```python
from build123d import *

# Parameters (mm, degrees)
SKETCH1_W                    = 406.4
SKETCH1_H                    = 50.8
EXTRUDE1_DEPTH               = 12.7
SKETCH2_W                    = 12.7
SKETCH2_H                    = 50.8
CUT_EXTRUDE1_DEPTH           = 3.175
SKETCH3_W                    = 44.45
SKETCH3_H                    = 31.75
SKETCH3_W_2                  = 76.2
CUT_EXTRUDE2_DEPTH           = 9.525
FILLET1_R                    = 6.35
SKETCH4_R                    = 2.38125
CUT_EXTRUDE3_DEPTH           = 15.875
SKETCH5_R                    = 3.175
CUT_EXTRUDE4_DEPTH           = 410.673437783
SKETCH6_R                    = 6.7437
CUT_EXTRUDE5_DEPTH           = 410.759551445
CUT_EXTRUDE5_DRAFT           = -41
CUT_EXTRUDE5_PROFILE_2_DEPTH = 410.759551445
CUT_EXTRUDE5_PROFILE_2_DRAFT = -41
CUT_EXTRUDE5_PROFILE_3_DEPTH = 410.759551445
CUT_EXTRUDE5_PROFILE_3_DRAFT = -41
CUT_EXTRUDE5_PROFILE_4_DEPTH = 410.759551445
CUT_EXTRUDE5_PROFILE_4_DRAFT = -41
SKETCH7_R                    = 3.175
CUT_EXTRUDE6_DEPTH           = 15.875
CUT_EXTRUDE7_START           = -15.875
SKETCH8_R                    = 3.175
CUT_EXTRUDE7_DEPTH           = 15.875


with BuildPart() as part:
    # Sketch1 → Extrude1 (new body)
    with BuildSketch(Plane(origin=(0, 0, 0), x_dir=(0, 0, -1), z_dir=(1, 0, 0))):
        with Locations((-203.2, 25.4)):
            Rectangle(SKETCH1_W, SKETCH1_H)
    extrude(amount=EXTRUDE1_DEPTH)

    # Sketch2 → Cut-Extrude1 (cut)
    with BuildSketch(Plane.ZY):
        with Locations((146.05, 25.4)):
            Rectangle(SKETCH2_W, SKETCH2_H)
        with Locations((260.35, 25.4)):
            Rectangle(SKETCH2_W, SKETCH2_H)
    extrude(amount=-CUT_EXTRUDE1_DEPTH, mode=Mode.SUBTRACT)

    # Sketch3 → Cut-Extrude2 (cut)
    with BuildSketch(Plane.ZY):
        with Locations((47.625, 25.4)):
            Rectangle(SKETCH3_W, SKETCH3_H)
        with Locations((104.775, 25.4)):
            Rectangle(SKETCH3_W, SKETCH3_H)
        with Locations((203.2, 25.4)):
            Rectangle(SKETCH3_W_2, SKETCH3_H)
        with Locations((301.625, 25.4)):
            Rectangle(SKETCH3_W, SKETCH3_H)
        with Locations((358.775, 25.4)):
            Rectangle(SKETCH3_W, SKETCH3_H)
    extrude(amount=-CUT_EXTRUDE2_DEPTH, mode=Mode.SUBTRACT)

    # Fillet1
    fillet1_edges = [part.edges().sort_by_distance(p)[0] for p in [
        (4.7625, 9.525, 25.4),
        (4.7625, 41.275, 25.4),
        (4.7625, 41.275, 69.85),
        (4.7625, 9.525, 69.85),
        (4.7625, 41.275, 127),
        (4.7625, 9.525, 127),
        (4.7625, 9.525, 82.55),
        (4.7625, 41.275, 82.55),
        (4.7625, 9.525, 165.1),
        (4.7625, 41.275, 165.1),
        (4.7625, 41.275, 241.3),
        (4.7625, 9.525, 241.3),
        (4.7625, 9.525, 279.4),
        (4.7625, 41.275, 279.4),
        (4.7625, 41.275, 323.85),
        (4.7625, 9.525, 323.85),
        (4.7625, 9.525, 336.55),
        (4.7625, 41.275, 336.55),
        (4.7625, 41.275, 381),
        (4.7625, 9.525, 381),
    ]]
    fillet(fillet1_edges, radius=FILLET1_R)

    # Sketch4 → Cut-Extrude3 (cut)
    with BuildSketch(Plane(origin=(0, 50.8, 0), x_dir=(-1, 0, 0), z_dir=(0, 1, 0))):
        with Locations(Location((-6.35, 19.05, 0), (0, 0, 90))):
            Circle(SKETCH4_R)
        with Locations(Location((-6.35, 133.35, 0), (0, 0, 90))):
            Circle(SKETCH4_R)
        with Locations(Location((-6.35, 273.05, 0), (0, 0, 90))):
            Circle(SKETCH4_R)
        with Locations(Location((-6.35, 387.35, 0), (0, 0, 90))):
            Circle(SKETCH4_R)
    cut_extrude3 = extrude(amount=-CUT_EXTRUDE3_DEPTH, mode=Mode.SUBTRACT)

    # Mirror1: Cut-Extrude3 across plane
    add(cut_extrude3.mirror(Plane.ZX.offset(25.4)), mode=Mode.SUBTRACT)

    # Sketch5 → Cut-Extrude4 (cut, through all)
    with BuildSketch(Plane.ZY.offset(-3.175)):
        with Locations((260.35, 41.275)):
            Circle(SKETCH5_R)
        with Locations((260.35, 9.525)):
            Circle(SKETCH5_R)
        with Locations((146.05, 41.275)):
            Circle(SKETCH5_R)
        with Locations((146.05, 9.525)):
            Circle(SKETCH5_R)
    extrude(amount=-CUT_EXTRUDE4_DEPTH, mode=Mode.SUBTRACT)


with BuildPart() as cut_extrude5_tool:
    # Sketch6 → Cut-Extrude5 (with draft: the straight prism first)
    with BuildSketch(Plane(origin=(12.7, 0, 0), x_dir=(0, 0, -1), z_dir=(1, 0, 0))):
        with Locations((-260.35, 41.275)):
            Circle(SKETCH6_R)
    extrude(amount=-CUT_EXTRUDE5_DEPTH)
    # Cut-Extrude5: the draft: its side faces are tilted about the plane it starts from
    cut_extrude5_sides = [cut_extrude5_tool.faces().sort_by_distance(p)[0] for p in [
        (-192.679775722, 41.275, 267.0937),
    ]]
    draft(cut_extrude5_sides, Plane(origin=(12.7, 0, 0), x_dir=(0, 0, -1), z_dir=(1, 0, 0)), CUT_EXTRUDE5_DRAFT)


with BuildPart() as part_1:
    add(part.part)

    # Cut-Extrude5: cut by cut_extrude5_tool
    add(cut_extrude5_tool.part, mode=Mode.SUBTRACT)


with BuildPart() as cut_extrude5_profile_2_tool:
    # Sketch6 → Cut-Extrude5 profile 2 (with draft: the straight prism first)
    with BuildSketch(Plane(origin=(12.7, 0, 0), x_dir=(0, 0, -1), z_dir=(1, 0, 0))):
        with Locations((-260.35, 9.525)):
            Circle(SKETCH6_R)
    extrude(amount=-CUT_EXTRUDE5_PROFILE_2_DEPTH)
    # Cut-Extrude5 profile 2: the draft: its side faces are tilted about the plane it starts from
    cut_extrude5_profile_2_sides = [cut_extrude5_profile_2_tool.faces().sort_by_distance(p)[0] for p in [
        (-192.679775722, 9.525, 267.0937),
    ]]
    draft(cut_extrude5_profile_2_sides, Plane(origin=(12.7, 0, 0), x_dir=(0, 0, -1), z_dir=(1, 0, 0)), CUT_EXTRUDE5_PROFILE_2_DRAFT)


with BuildPart() as part_2:
    add(part_1.part)

    # Cut-Extrude5 profile 2: cut by cut_extrude5_profile_2_tool
    add(cut_extrude5_profile_2_tool.part, mode=Mode.SUBTRACT)


with BuildPart() as cut_extrude5_profile_3_tool:
    # Sketch6 → Cut-Extrude5 profile 3 (with draft: the straight prism first)
    with BuildSketch(Plane(origin=(12.7, 0, 0), x_dir=(0, 0, -1), z_dir=(1, 0, 0))):
        with Locations((-146.05, 9.525)):
            Circle(SKETCH6_R)
    extrude(amount=-CUT_EXTRUDE5_PROFILE_3_DEPTH)
    # Cut-Extrude5 profile 3: the draft: its side faces are tilted about the plane it starts from
    cut_extrude5_profile_3_sides = [cut_extrude5_profile_3_tool.faces().sort_by_distance(p)[0] for p in [
        (-192.679775722, 9.525, 152.7937),
    ]]
    draft(cut_extrude5_profile_3_sides, Plane(origin=(12.7, 0, 0), x_dir=(0, 0, -1), z_dir=(1, 0, 0)), CUT_EXTRUDE5_PROFILE_3_DRAFT)


with BuildPart() as part_3:
    add(part_2.part)

    # Cut-Extrude5 profile 3: cut by cut_extrude5_profile_3_tool
    add(cut_extrude5_profile_3_tool.part, mode=Mode.SUBTRACT)


with BuildPart() as cut_extrude5_profile_4_tool:
    # Sketch6 → Cut-Extrude5 profile 4 (with draft: the straight prism first)
    with BuildSketch(Plane(origin=(12.7, 0, 0), x_dir=(0, 0, -1), z_dir=(1, 0, 0))):
        with Locations((-146.05, 41.275)):
            Circle(SKETCH6_R)
    extrude(amount=-CUT_EXTRUDE5_PROFILE_4_DEPTH)
    # Cut-Extrude5 profile 4: the draft: its side faces are tilted about the plane it starts from
    cut_extrude5_profile_4_sides = [cut_extrude5_profile_4_tool.faces().sort_by_distance(p)[0] for p in [
        (-192.679775722, 41.275, 152.7937),
    ]]
    draft(cut_extrude5_profile_4_sides, Plane(origin=(12.7, 0, 0), x_dir=(0, 0, -1), z_dir=(1, 0, 0)), CUT_EXTRUDE5_PROFILE_4_DRAFT)


with BuildPart() as part_4:
    add(part_3.part)

    # Cut-Extrude5 profile 4: cut by cut_extrude5_profile_4_tool
    add(cut_extrude5_profile_4_tool.part, mode=Mode.SUBTRACT)

    # Sketch7 → Cut-Extrude6 (cut)
    with BuildSketch(Plane(origin=(0, 0, 0), x_dir=(-1, 0, 0), z_dir=(0, 0, -1))):
        with Locations((-6.35, 41.275)):
            Circle(SKETCH7_R)
        with Locations((-6.35, 9.525)):
            Circle(SKETCH7_R)
    extrude(amount=-CUT_EXTRUDE6_DEPTH, mode=Mode.SUBTRACT)

    # Sketch8 → Cut-Extrude7 (cut)
    with BuildSketch(Plane.XY.offset(406.4).offset(CUT_EXTRUDE7_START)):
        with Locations(Location((6.35, 41.275, 0), (0, 0, 180))):
            Circle(SKETCH8_R)
        with Locations(Location((6.35, 9.525, 0), (0, 0, 180))):
            Circle(SKETCH8_R)
    extrude(amount=CUT_EXTRUDE7_DEPTH, mode=Mode.SUBTRACT)


solid = part_4.part
```
Build history of the part. All positions in model axes, mm. A direction names the side the tool comes from. Round coordinates to 2 decimals unless told otherwise and drop trailing zeros. Write each loop counter-clockwise with the first axis right and the second up, starting at its lowest first coordinate (ties: lowest second). Pieces come first, ordered by that corner, then holes. Notation, with made-up numbers: (14, 38) -> (58, 38) arc R23 cw to (58, 66) -> close; hole circle Ø7 at (-31, 40). An arc over 180 degrees is marked (long way). Put each result on its own line as item: value.
Item 1: Slice it at B-B, the plane z = 98.5. Give the cut face in (x, y) (3 decimals).
Here are the results:
outline: (0, 0) -> (12.7, 0) -> (12.7, 50.8) -> (0, 50.8) -> (0, 41.275) -> (9.525, 41.275) -> (9.525, 9.525) -> (0, 9.525) -> close
Item 2: Wall check: probe 1 along Z at (x, y) = (4.5, 25); probe 2 along Y at (x, z) = (7.25, 146.05); probe 3 along Z at (x, y) = (5.75, 48.5). Give the ranges that are in metal, low to high. Write a range as from..to.
Here are the results:
probe 1: z = 0..25.4, 69.85..82.55, 127..165.1, 241.3..279.4, 323.85..336.55, 381..406.4
probe 2: y = 0..6.35, 12.7..38.1, 44.45..50.8
probe 3: z = 0..16.75, 21.35..131.05, 135.65..270.75, 275.35..385.05, 389.65..406.4
Item 3: Two-plate mould, pull along X, no slides. Class faces 1 (the face through (6, 25, 406.4)), 2 (the face through (6, 41, 390.525)), 3 (the face through (8.851, 39.973, 142.911)), 4 (the face through (6, 9, 390.525)): pulls with the +X half, pulls with the -X half, needs draft (parallel to the pull), parting line crosses it, or undercut.
Here are the results:
face 1: needs draft
face 2: undercut
face 3: pulls with the +X half
face 4: undercut
Item 4: Tool access for faces 5 (the face through (3.175, 26, 146)), 6 (the face through (6, 10, 15.875)), 7 (the face through (5.847, 9.665, 257.178)), 8 (the face through (5, 9.525, 47)): list every direction of +Z, -Z, +X, -X, +Y, -Y with a clear straight run to the whole face (end or side of a thin tool).
Here are the results:
face 5: -X, +Y, -Y
face 6: -Z
face 7: +X, -X
face 8: -X
Item 5: Flat gauge pins, fed straight in: P1, Ø6, axis at x = 6.5, z = 45.5, coming from the -Y side; P2, Ø1.4, axis at x = 7.5, z = 273, coming from the -Y side (3 decimals); P3, Ø5.5, axis at x = 6.35, y = 41.275, coming from the -Z side (3 decimals). Where does each tip first touch, or does it go through?
Here are the results:
P1: stops at y = 0
P2: stops at y = 15.875
P3: stops at z = 15.875
